Job drawing, mm, ordinate dimensions from the low corner. One solid piece. A direction names the side the tool comes from. Round coordinates to 2 decimals unless told otherwise and drop trailing zeros. Loops run counter-clockwise (first coordinate to the right, second up) from the corner with the lowest first, then second, coordinate; pieces in that order, holes last.
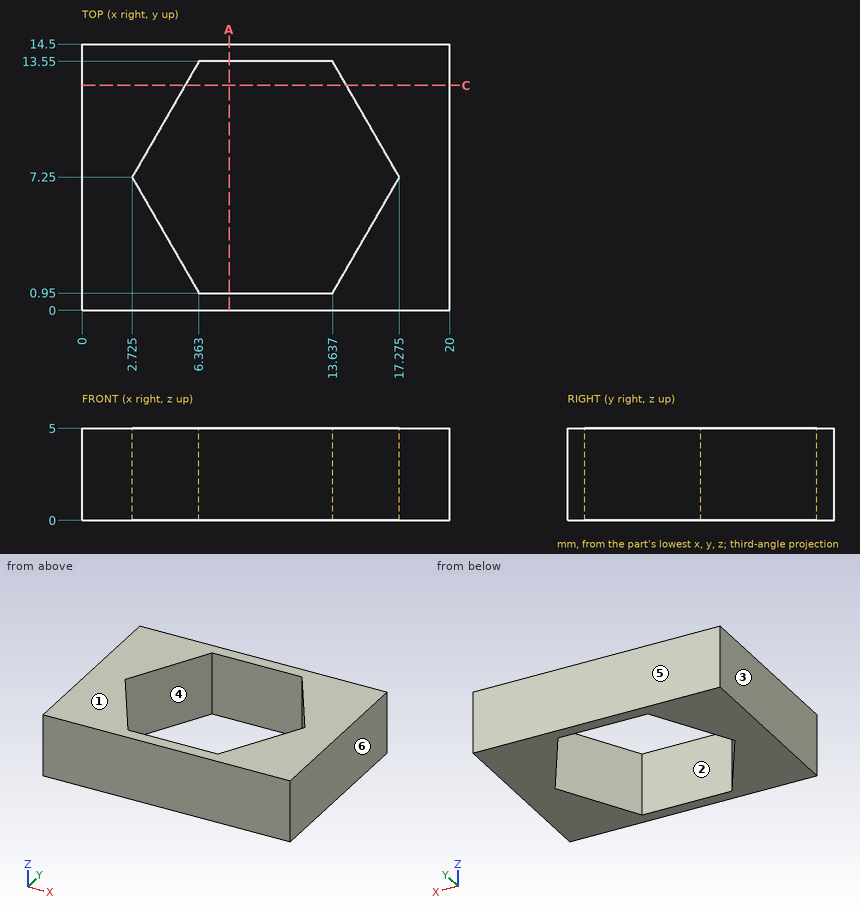
1) Tool access for the marked faces 1 and 2: list every direction of +Z, -Z, +X, -X, +Y, -Y with a clear straight run to the whole face (end or side of a thin tool).
Values:
face 1: +Z, +X, -X, +Y, -Y
face 2: +Z, -Z
2) Slice it at A-A, the plane x = 8. Give the cut face in (y, z).
Values:
outline: (0, 0) - (0.95, 0) - (0.95, 5) - (0, 5) - close; (13.55, 0) - (14.5, 0) - (14.5, 5) - (13.55, 5) - close
3) Mould opens along X. For the marked faces 3, 4, 5 and 6 say: released by +X, released by -X, zero draft, split by the parting line, or undercut.
Values:
face 3: released by -X
face 4: undercut
face 5: zero draft
face 6: released by +X
4) Wall check: line 1 along Y through (x, z) = (9.5, 3.95); line 2 along X through (y, z) = (13, 3.7) (1 decimal); line 3 along X through (y, z) = (12.25, 2.9). Give the ranges that are in metal, low to high.
Values:
line 1: y = 0 to 0.95, 13.55 to 14.5
line 2: x = 0 to 6, 14 to 20
line 3: x = 0 to 5.61, 14.39 to 20
5) Slice it at C-C, the plane y = 12.25. Give the cut face in (x, z).
Values:
outline: (0, 0) - (5.61, 0) - (5.61, 5) - (0, 5) - close; (14.39, 0) - (20, 0) - (20, 5) - (14.39, 5) - close
